from build123d import *

# Parameters (mm, degrees)
F0_W     = 57.3121234775
F0_H     = 25.3932457417
F1_DEPTH = 38.1
F3_DEPTH = 12.7
F5_DEPTH = 12.7
F7_DEPTH = 12.7


with BuildPart() as f1:
    # F0 (on Front) → F1 (new body)
    with BuildSketch(Plane.XZ):
        with Locations((26.2444131076, 12.6966228709)):
            Rectangle(F0_W, F0_H)
    extrude(amount=F1_DEPTH)

    # F2 (on face) → F3 (cut)
    with BuildSketch(Plane.XZ.offset(38.1)):
        Polygon((54.9004748464, 25.3932457417), (16.6383513689, 25.3932457417), (29.3653700501, 0), (54.9004748464, 0), align=None)
    extrude(amount=-F3_DEPTH, mode=Mode.SUBTRACT)

    # F4 (on face) → F5 (cut)
    with BuildSketch(Plane.XZ.offset(25.4)):
        Polygon((54.9004748464, 0), (54.9004748464, 25.3932457417), (42.4166470766, 25.3932457417), align=None)
    extrude(amount=-F5_DEPTH, mode=Mode.SUBTRACT)

    # F6 (on face) → F7 (cut)
    with BuildSketch(Plane(origin=(0, 0, 0), x_dir=(-1, 0, 0), z_dir=(0, 1, 0))):
        Polygon((-29.3199047446, 0), (-16.6687499732, 25.3932457417), (-54.9004748464, 25.3932457417), (-54.9004748464, 0), (-42.1420186758, 0), align=None)
    extrude(amount=-F7_DEPTH, mode=Mode.SUBTRACT)


solid = f1.part
Geometry: final body of the model. Coordinates: model frame, mm. A direction names the side the tool comes from. Give positions to 0.01 mm unless a question says otherwise; leave off trailing zeros. Write each loop counter-clockwise with the first axis right and the second up, starting at its lowest first coordinate (ties: lowest second). Pieces come first, ordered by that corner, then holes. Notation, with made-up numbers: (18.5, -26.75) - (59.5, -26.75) arc R29 cw to (59.5, 11.25) - close; hole circle Ø1 at (29, 77.25). An arc over 180 degrees is marked (long way). Return JSON: item names as keys, results as strings. Group by question number.
1) Section D-D on z = 21.25. Return the cut outline in (x, y), plus the area to 3 significant figures.
2) Section B-B on x = 35. Return the cut outline in (y, z), plus the area to 3 significant figures.
3) First-contact query: P1, Ø1.5, axis at x = 44.5, z = 8, coming from the -Y side; P2, Ø1, axis at x = 41, z = 10.5, coming from the +Y side; P3, Ø8, axis at y = -13.5, z = 7.5, coming from the +X side. Flat tips, straight axial feed; report the tip coordinate or a pass-through.
4) Set-up query: faces 1 (the flat face through (36, -25.4, 13)), 2 (the flat face through (48.571, -19.139, 12.874)), 3 (the flat face through (36, -12.7, 13)). Return all of +Z, -Z, +X, -X, +Y, -Y with unobstructed straight access to the full face (end or side cutting, diameter ignored); none if empty.
5) Section A-A on z = 14.75. Return the cut outline in (x, y).
6) Section C-C on y = -29. Return the cut outline in (x, z), plus the area to 3 significant figures.
7) Line query: line 1 (Y direction, x = 35, z = 12.25); line 2 (X direction, y = -19.5, z = 19.75); line 3 (X direction, y = -9, z = 9.25). Output: solid intervals per line, ascending.
Filled in:
{
 "1": {"outline": "(-2.41, -38.1) - (18.71, -38.1) - (18.71, -25.4) - (44.45, -25.4) - (44.45, -12.7) - (18.73, -12.7) - (18.73, 0) - (-2.41, 0) - close", "area": "1,130 mm^2"},
 "2": {"outline": "(-25.4, 0) - (-12.7, 0) - (-12.7, 25.39) - (-25.4, 25.39) - close", "area": "322 mm^2"},
 "3": {"P1": "stops at y = -25.4", "P2": "stops at y = -12.7", "P3": "stops at x = 53.18"},
 "4": {"face 1": "+Z, +X, -Y", "face 2": "+Z, +X, +Y, -Y", "face 3": "+Z, +X, +Y"},
 "5": {"outline": "(-2.41, -38.1) - (21.97, -38.1) - (21.97, -25.4) - (47.65, -25.4) - (47.65, -12.7) - (21.97, -12.7) - (21.97, 0) - (-2.41, 0) - close"},
 "6": {"outline": "(-2.41, 0) - (29.37, 0) - (16.64, 25.39) - (-2.41, 25.39) - close", "area": "645 mm^2"},
 "7": {"line 1": "y = -25.4 to -12.7", "line 2": "x = -2.41 to 45.19", "line 3": "x = -2.41 to 24.71"}
}
